Design review of the part built by this model. Coordinates are the model's own, in mm. A direction names the side the tool comes from. Coordinates: 2 decimals unless noted, no trailing zeros. Write each loop counter-clockwise with the first axis right and the second up, starting at its lowest first coordinate (ties: lowest second). Pieces come first, ordered by that corner, then holes. Notation, with made-up numbers: M 38.5,83 L 68.5,83 A14 ccw 68.5,92 Z; hole C 21,26.25 d9. An arc over 180 degrees is marked long. Write each question's results on one line, items separated by ' | '. Start each with the question number.
Autodesk Inventor part; units mm, degrees
ref_plane "YZ Plane" through (0, 0, 0) normal (1, 0, 0) x (0, 1, 0)
ref_plane "XZ Plane" through (0, 0, 0) normal (0, 1, 0) x (-1, 0, 0)
ref_plane "XY Plane" through (0, 0, 0) normal (0, 0, 1) x (1, 0, 0)
sketch "Sketch1" plane through (0, 0, 0) normal (0, 1, 0) x (-1, 0, 0)
  circle A0 centre (0, 0) radius 4.75
  dimension "d0" = 9.5
extrude "Extrusion1" add sketch "Sketch1" along normal blind 17.5
sketch "Sketch2" plane through (0, 17.5, 0) normal (0, 1, 0) x (1, 0, 0)
  circle A0 centre (0, 0) radius 8
  dimension "d3" = 16
extrude "Extrusion2" add sketch "Sketch2" along normal blind 17
sketch "Sketch3" plane through (0, 0, 0) normal (0, 0, 1) x (1, 0, 0)
  line L0 (0, 39.2) -> (0, 22.5)
  line L1 (0, 22.5) -> (10, 39.2)
  line L2 (10, 39.2) -> (0, 39.2)
  line L3 (8, 17.5) -> (-8, 17.5)
  line L4 (0, -7.84) -> (0, 47.04)
  point P0 (0, 0)
  dimension "d6" = 5
  dimension "d7" = 10
  dimension "d8" = 16.7
revolve "Revolution1" cut sketch "Sketch3" angle 360 about axis through (0, -10, 0) along (0, 1, 0)
sketch "Sketch4" plane through (0, 34.5, 0) normal (0, 1, 0) x (1, 0, 0)
  circle A0 centre (0, 0) radius 5
  dimension "d10" = 10
extrude "Extrusion3" cut sketch "Sketch4" against normal blind 12.1
sketch "Sketch5" plane through (0, 34.5, 0) normal (0, 1, 0) x (1, 0, 0)
  line L0 (-8.5, -2.25) -> (8.5, -2.25)
  line L1 (8.5, -2.25) -> (8.5, 2.25)
  line L2 (8.5, 2.25) -> (-8.5, 2.25)
  line L3 (-8.5, 2.25) -> (-8.5, -2.25)
  line L4 (-8.5, -2.25) -> (8.5, 2.25) construction
  line L5 (8.5, -2.25) -> (-8.5, 2.25) construction
  point P0 (0, 0)
  dimension "d13" = 17
  dimension "d14" = 4.5
extrude "Extrusion4" cut sketch "Sketch5" against normal blind 12
sketch "Sketch6" plane through (6.8243, 34.5, -2.25) normal (0, 0, 1) x (1, 0, 0)
  line L0 (-13.6486, 0) -> (0, 0)
  line L1 (-11.2894, -3.65) -> (-2.3591, -3.65)
  line L2 (0, 0) -> (0, -3.5) construction
  point P0 (-6.8243, -34.5)
  dimension "d17" = 3.65
  dimension "d18" = 2.3591
sketch "Sketch9" plane through (0, 22.4, 0) normal (0, 1, 0) x (1, 0, 0)
  circle A0 centre (0, 0) radius 5
  arc A1 (0, -5) -> (0, 5) centre (0, 0) ccw
  line L0 (0, 0) -> (0, -5) construction
  line L1 (0, 0) -> (0, 5) construction
  line L2 (0, 5) -> (0, -5)
  dimension "d19" = 180
revolve "Revolution2" cut sketch "Sketch9" angle 360 about axis through (0, 22.4, 0) along (0, 0, -1) picked at (1.0391, 1.3031) contours A0 L2
sketch "Sketch16" plane through (0, 0, 0) normal (0, -1, 0) x (1, 0, 0)
  arc A0 (1.7108, -2.525) -> (-1.7108, -2.525) centre (0, 0) ccw
  line L0 (1.7108, -2.525) -> (-1.7108, -2.525)
  dimension "d55" = 6.1
  dimension "d56" = 0.525
extrude "Extrusion8" cut sketch "Sketch16" against normal blind 12
properties part number "shaft"
Item 1: Insertion check: pin 1 Ø2.5 at (x, y) = (0, 7.5) entering from +Z; pin 2 Ø2 at (y, z) = (5, -2) entering from -X; pin 3 Ø2 at (x, y) = (2.5, 29) entering from +Z; pin 4 Ø2 at (x, y) = (-6.5, 15) entering from -Z. Each pin has a flat end and moves straight along its axis. Give the tip position at first contact, or say it passes through.
Item 2: For faces 1 (the flat face through (6, 29, -2.25)), 2 (the cylindrical face through (7.39, 25.88, -3.06)), 3 (the flat face through (0, 17.5, 5)), 4 (the flat face through (0, 34.5, 7.5)), 5 (the conical face through (-0.1, 31.89, 5.62)), list the 3-axis set-ups (+Z, -Z, +X, -X, +Y, -Y) from which the entire face can be reached by the end or side of a thin tool; tool diameter is ignored.
Item 3: We need section D-D on y = 4.5. State the section outline as (x, z) points (3 decimals).
Item 4: We need section B-B on x = 0. State the section outline as (y, z) points (3 decimals), then the cut area to 3 significant figures.
Item 5: We need section A-A on y = 24. State the section outline as (x, z) points, then the cut area to 3 significant figures.
Item 6: Draft analysis for pull direction X (two halves, no side actions). For faces 6 (the cylindrical face through (-2.192, 8.628, 4.214)), 7 (the conical face through (0.1, 31.89, -5.62)), 8 (the flat face through (0, 0, -3)), state which applies: released by +X, released by -X, zero draft, split by the parting line, or undercut.
Item 7: We need section C-C on z = 0. State the section outline as (x, y) points.
Item 8: Wall thickness on L1, parallel to Z at x = 0, y = 24; L2, parallel to Z at x = 3.25, y = 29; L3, parallel to Y at x = 6.25, z = -4.5: over which ranges is each line inside the solid? List them lowest first.
Answer:
1) pin 1: stops at z = 4.75 | pin 2: stops at x = -4.64 | pin 3: stops at z = 7.86 | pin 4: passes through
2) face 1: +X, -X, +Y | face 2: +Y, -Y | face 3: -Y | face 4: +Z, -Z, +X, -X, +Y | face 5: +Y
3) outline: C 0,0 d9.5; hole M -1.711,-2.525 L 1.711,-2.525 A3.05 ccw long Z
4) outline: M 0,-4.75 L 17.5,-4.75 L 17.5,-8 L 34.5,-8 L 34.5,-7.186 L 30.85,-5 L 22.4,-5 A5 cw 22.4,5 L 30.85,5 L 34.5,7.186 L 34.5,8 L 17.5,8 L 17.5,4.75 L 0,4.75 L 0,3.05 L 12,3.05 L 12,-2.525 L 0,-2.525 Z | area: 203 mm^2
5) outline: M -7.68,-2.25 A8 ccw 7.68,-2.25 L 4.47,-2.25 A5 cw -4.47,-2.25 Z; M -7.68,2.25 L -4.47,2.25 A5 cw 4.47,2.25 L 7.68,2.25 A8 ccw Z | area: 94.9 mm^2
6) face 6: split by the parting line | face 7: undercut | face 8: zero draft
7) outline: M -8,17.5 L -4.75,17.5 L -4.75,0 L -3.05,0 L -3.05,12 L 3.05,12 L 3.05,0 L 4.75,0 L 4.75,17.5 L 8,17.5 L 8,22.5 L 5,22.5 L 5,22.4 A5 cw -5,22.4 L -5,22.5 L -8,22.5 Z
8) L1: z = -8 to -5, 5 to 8 | L2: z = -7.31 to -3.8, 3.8 to 7.31 | L3: y = 17.5 to 34.5
